For this review, take the finished solid that the model builds, in its own axes (mm). A direction names the side the tool comes from. Give positions to 0.01 mm unless a question says otherwise; leave off trailing zeros. Order: outer loops, then holes, each group sorted by start corner. A loop starts at its lowest first (then second) coordinate and runs counter-clockwise, first axis right, second up. Notation, with made-up numbers: (63, 86.5) -> (70, 86.5) arc R16 ccw to (70, 96.5) -> close; hole circle Ø1 at (51, 11). An arc over 180 degrees is marked (long way). Return JSON: item names as keys, results as strings. Group by question number.
1) For faces 5 (the face through (0, 15, -28)), 6 (the face through (-10.99, 0.99, 8.67)), 7 (the face through (-17, 11, 0)), 8 (the face through (-3, 1, 7)), list the 3-axis set-ups (+Z, -Z, +X, -X, +Y, -Y) from which the entire face can be reached by the end or side of a thin tool; tool diameter is ignored.
2) Add section B-B (z = -35). Give the boundary of the cut face in (x, y), then the cut area to 3 significant figures.
3) To check wall thickness, follow line 1 along Y through (x, z) = (-4, -10); line 2 along Y through (x, z) = (-2.5, -11); line 3 along X through (y, z) = (-3.5, -17). State the ranges of each line that lie inside material, in increasing order.
4) The part is to be moulded in two halves that separate along X. For faces 1 (the face through (0, -25, -12)), 2 (the face through (0, -25, -14)), 3 (the face through (-25, -51, -15)), 4 (the face through (1, 32, 4)), say which applies: released by +X, released by -X, zero draft, split by the parting line, or undercut.
5) Add section A-A (y = -5.5). Give the boundary of the cut face in (x, z).
6) Add section C-C (x = 16). Give the boundary of the cut face in (y, z), then the cut area to 3 significant figures.
7) Insertion check: P1, Ø4, axis at x = 0.5, z = -28, coming from the +Y side; P2, Ø1.6, axis at x = -3.5, y = 37.5, coming from the -Z side; P3, Ø8, axis at y = -10, z = -25.5, coming from the +X side. Each pin has a flat end and moves straight along its axis. Give the tip position at first contact, or say it passes through.
from build123d import *

# Parameters (mm, degrees)
MOTOR_FRONTPLATE_DEPTH           = 2
MOTORKRYBBE_START                = 50
MOTORKRYBBE_DEPTH                = 50
SKYGGE_KAPPE_DEPTH               = 8
SKYGGE_TOPP_DEPTH                = 2
LEDHOLDER_TOPP_DEPTH             = 13
LEDHOLDER_START                  = 13
LEDHOLDER_BUNN_DEPTH             = 13
SKETCH10_R                       = 2.5
LEDHULL_DEPTH                    = 51.950956811
ROTORKAPPE_VEGG_DEPTH            = 20
SKETCH12_R                       = 13
LASERHOLDER_DEPTH                = 4
LASER_HULL_D                     = 6
BUNNPLATE_DEPTH                  = 2
BOSS_EXTRUDE12_DEPTH             = 5
BOSS_EXTRUDE12_DIRECTION_2_REACH = 72.207
LED_START                        = -38
LED_KABELHOLDER_DEPTH            = 38
KABELHOLDER_HULL_REACH           = 73.729
FILLET1_R                        = 5
BOSS_EXTRUDE14_DEPTH             = 5


with BuildPart() as part:
    # Sketch1 → Motor-frontplate (new body)
    with BuildSketch(Plane(origin=(0, 0, 0), x_dir=(1, 0, 0), z_dir=(0, 1, 0))):
        with BuildLine():
            ThreePointArc((-3, 0), (0, 3), (3, 0))
            Line((3, 0), (3, -13.674794331))
            ThreePointArc((3, -13.674794331), (10.908712115, -8.774964387), (14, 0))
            ThreePointArc((14, 0), (0, 14), (-14, 0))
            ThreePointArc((-14, 0), (-10.908712115, -8.774964387), (-3, -13.674794331))
            Line((-3, -13.674794331), (-3, 0))
        make_face()
        with BuildLine():
            Line((14, 0), (24, 0))
            ThreePointArc((24, 0), (0, 24), (-24, 0))
            Line((-24, 0), (-14, 0))
            ThreePointArc((-14, 0), (0, 14), (14, 0))
        make_face()
    extrude(amount=MOTOR_FRONTPLATE_DEPTH)

    # Sketch2 → Motorkrybbe (add)
    with BuildSketch(Plane.XZ.offset(MOTORKRYBBE_START)):
        with BuildLine():
            Line((-12, 0), (-14, 0))
            ThreePointArc((-14, 0), (0, -14), (14, 0))
            Line((14, 0), (12, 0))
            ThreePointArc((12, 0), (0, -12), (-12, 0))
        make_face()
    extrude(amount=-MOTORKRYBBE_DEPTH)

    # Sketch5 → Skygge - Kappe (add)
    with BuildSketch(Plane(origin=(0, 2, 0), x_dir=(1, 0, 0), z_dir=(0, 1, 0))):
        with BuildLine():
            Line((-24, 0), (-22, 0))
            ThreePointArc((-22, 0), (0, 22), (22, 0))
            Line((22, 0), (24, 0))
            ThreePointArc((24, 0), (0, 24), (-24, 0))
        make_face()
    extrude(amount=SKYGGE_KAPPE_DEPTH)

    # Sketch6 → Skygge - Topp (add)
    with BuildSketch(Plane(origin=(0, 10, 0), x_dir=(1, 0, 0), z_dir=(0, 1, 0))):
        with BuildLine():
            Line((-24, 0), (-11, 0))
            ThreePointArc((-11, 0), (0, 11), (11, 0))
            Line((11, 0), (24, 0))
            ThreePointArc((24, 0), (0, 24), (-24, 0))
        make_face()
    extrude(amount=SKYGGE_TOPP_DEPTH)

    # Sketch7 → LEDholder - Topp (add)
    with BuildSketch(Plane(origin=(0, 12, 0), x_dir=(1, 0, 0), z_dir=(0, 1, 0))):
        with BuildLine():
            Line((-4, 12.369316877), (-4, 23.664319132))
            ThreePointArc((-4, 23.664319132), (0, 24), (4, 23.664319132))
            Line((4, 23.664319132), (4, 12.369316877))
            ThreePointArc((4, 12.369316877), (0, 13), (-4, 12.369316877))
        make_face()
    extrude(amount=LEDHOLDER_TOPP_DEPTH)

    # Sketch8 → LEDholder - Bunn (add)
    with BuildSketch(Plane.XZ.offset(LEDHOLDER_START)):
        with BuildLine():
            ThreePointArc((-4, -23.664319132), (0, -24), (4, -23.664319132))
            Line((4, -23.664319132), (4, -13.416407865))
            ThreePointArc((4, -13.416407865), (0, -14), (-4, -13.416407865))
            Line((-4, -13.416407865), (-4, -23.664319132))
        make_face()
    extrude(amount=-LEDHOLDER_BUNN_DEPTH)

    # Sketch10 → LEDhull (cut, through all)
    with BuildSketch(Plane.XZ.offset(13)):
        with Locations(Location((0, -17, 0), (0, 0, 270))):
            Circle(SKETCH10_R)
    extrude(amount=-LEDHULL_DEPTH, mode=Mode.SUBTRACT)

    # Sketch11 → Rotorkappe - Vegg (add)
    with BuildSketch(Plane(origin=(0, 12, 0), x_dir=(1, 0, 0), z_dir=(0, 1, 0))):
        with BuildLine():
            Line((-13, 0), (-11, 0))
            ThreePointArc((-11, 0), (0, 11), (11, 0))
            Line((11, 0), (13, 0))
            ThreePointArc((13, 0), (0, 13), (-13, 0))
        make_face()
    extrude(amount=ROTORKAPPE_VEGG_DEPTH)

    # Sketch12 → Laserholder (add)
    with BuildSketch(Plane(origin=(0, 32, 0), x_dir=(1, 0, 0), z_dir=(0, 1, 0))):
        with Locations(Location((0, 0, 0), (0, 0, 107.920213139))):
            Circle(SKETCH12_R)
    extrude(amount=LASERHOLDER_DEPTH)

    # Laser - hull (through all)
    with Locations(Plane(origin=(0, 36, 0), x_dir=(1, 0, 0), z_dir=(0, 1, 0))):
        with Locations((0, 0)):
            Hole(LASER_HULL_D / 2)

    # Sketch16 → Bunnplate (add)
    with BuildSketch(Plane.XZ.offset(50)):
        with BuildLine():
            Line((-17, -40), (17, -40))
            ThreePointArc((17, -40), (22.656854249, -37.656854249), (25, -32))
            Line((25, -32), (25, 2))
            ThreePointArc((25, 2), (22.656854249, 7.656854249), (17, 10))
            Line((17, 10), (-17, 10))
            ThreePointArc((-17, 10), (-22.656854249, 7.656854249), (-25, 2))
            Line((-25, 2), (-25, -32))
            ThreePointArc((-25, -32), (-22.656854249, -37.656854249), (-17, -40))
        make_face()
    extrude(amount=BUNNPLATE_DEPTH)

    # Sketch19 → Boss-Extrude12 (add)
    with BuildSketch(Plane.XY):
        Polygon((0, -33), (-5, -33), (-5, -30), (-7, -30), (-7, -35), (0, -35), align=None)
    boss_extrude12 = extrude(amount=BOSS_EXTRUDE12_DEPTH)

    # Sketch19 → Boss-Extrude12 direction 2 (add, up to next)
    with BuildSketch(Plane.XY, mode=Mode.PRIVATE) as boss_extrude12_direction_2_sk1:
        Polygon((0, -33), (-5, -33), (-5, -30), (-7, -30), (-7, -35), (0, -35), align=None)
    boss_extrude12_direction_2_tool1 = extrude(boss_extrude12_direction_2_sk1.sketch, amount=-BOSS_EXTRUDE12_DIRECTION_2_REACH, mode=Mode.PRIVATE) - part.part
    boss_extrude12_direction_2 = boss_extrude12_direction_2_tool1.solids().sort_by_distance((-4.25, -33.25, 0))[0]
    add(boss_extrude12_direction_2)

    # Mirror2: Boss-Extrude12, Boss-Extrude12 direction 2 across plane
    add(boss_extrude12.mirror(Plane(origin=(0, -35, -40.002), x_dir=(0, 0, 1), z_dir=(1, 0, 0))))
    add(boss_extrude12_direction_2.mirror(Plane(origin=(0, -35, -40.002), x_dir=(0, 0, 1), z_dir=(1, 0, 0))))

    # Sketch20 → LED - kabelholder (add)
    with BuildSketch(Plane(origin=(0, 25, 0), x_dir=(1, 0, 0), z_dir=(0, 1, 0)).offset(LED_START)):
        with BuildLine():
            Line((4, 23.664319132), (4, 38.664319132))
            Line((4, 38.664319132), (-4, 38.664319132))
            Line((-4, 38.664319132), (-4, 23.664319132))
            ThreePointArc((-4, 23.664319132), (0, 24), (4, 23.664319132))
        make_face()
    extrude(amount=LED_KABELHOLDER_DEPTH)

    # Sketch21 → Kabelholder - hull (cut, up to next)
    with BuildSketch(Plane(origin=(4, 0, 0), x_dir=(0, 0, -1), z_dir=(1, 0, 0)), mode=Mode.PRIVATE) as kabelholder_hull_sk1:
        with BuildLine():
            Line((25.664319132, 15), (30.664319132, 15))
            ThreePointArc((30.664319132, 15), (33.164319132, 17.5), (30.664319132, 20))
            Line((30.664319132, 20), (25.664319132, 20))
            ThreePointArc((25.664319132, 20), (23.164319132, 17.5), (25.664319132, 15))
        make_face()
    kabelholder_hull_tool1 = extrude(kabelholder_hull_sk1.sketch, amount=-KABELHOLDER_HULL_REACH, mode=Mode.PRIVATE) & part.part
    # Sketch21 → Kabelholder - hull (cut, up to next)
    with BuildSketch(Plane(origin=(4, 0, 0), x_dir=(0, 0, -1), z_dir=(1, 0, 0)), mode=Mode.PRIVATE) as kabelholder_hull_sk2:
        with BuildLine():
            ThreePointArc((30.664319132, -3), (33.164319132, -5.5), (30.664319132, -8))
            Line((30.664319132, -8), (25.664319132, -8))
            ThreePointArc((25.664319132, -8), (23.164319132, -5.5), (25.664319132, -3))
            Line((25.664319132, -3), (30.664319132, -3))
        make_face()
    kabelholder_hull_tool2 = extrude(kabelholder_hull_sk2.sketch, amount=-KABELHOLDER_HULL_REACH, mode=Mode.PRIVATE) & part.part
    add(kabelholder_hull_tool1.solids().sort_by_distance((4, 17.5, -28.164319))[0], mode=Mode.SUBTRACT)
    add(kabelholder_hull_tool2.solids().sort_by_distance((4, -5.5, -28.164319))[0], mode=Mode.SUBTRACT)

    # Fillet1
    fillet1_edges = [part.edges().sort_by_distance(p)[0] for p in [
        (0, -13, -38.664319132),
        (0, 25, -38.664319132),
    ]]
    fillet(fillet1_edges, radius=FILLET1_R)

    # Sketch22 → Boss-Extrude14 (add)
    with BuildSketch(Plane(origin=(0, 36, 0), x_dir=(1, 0, 0), z_dir=(0, 1, 0))):
        with BuildLine():
            Line((-3, 0), (-5, 0))
            ThreePointArc((-5, 0), (0, -5), (5, 0))
            Line((5, 0), (3, 0))
            ThreePointArc((3, 0), (0, -3), (-3, 0))
        make_face()
    extrude(amount=BOSS_EXTRUDE14_DEPTH)


solid = part.part
Evaluation:
{
 "1": {"face 5": "+X, -X", "face 6": "+Z, -X, +Y", "face 7": "+Z, -X", "face 8": "+Z"},
 "2": {"outline": "(-24.42, -52) -> (24.42, -52) -> (24.42, -50) -> (-24.42, -50) -> close; (-4, -12.82) -> (4, -12.82) -> (4, 24.82) -> (-4, 24.82) -> close", "area": "399 mm^2"},
 "3": {"line 1": "-52 to -50, -35 to -33, 0 to 2, 32 to 36", "line 2": "-52 to -50, -35 to -33, 0 to 2, 10 to 36", "line 3": "-4 to -2.5, 2.5 to 4"},
 "4": {"face 1": "undercut", "face 2": "split by the parting line", "face 3": "released by -X", "face 4": "undercut"},
 "5": {"outline": "(-14, 0) arc R14 ccw to (-4, -13.42) -> (-4, -23.16) -> (4, -23.16) -> (4, -13.42) arc R14 ccw to (14, 0) -> (12, 0) arc R12 cw to (-12, 0) -> close; (-4, -38.66) -> (4, -38.66) -> (4, -33.16) -> (-4, -33.16) -> close; hole circle Ø5 at (0, -17)"},
 "6": {"outline": "(-52, -40) -> (-50, -40) -> (-50, 10) -> (-52, 10) -> close; (0, -17.89) -> (12, -17.89) -> (12, 0) -> (10, 0) -> (10, -15.1) -> (2, -15.1) -> (2, 0) -> (0, 0) -> close", "area": "194 mm^2"},
 "7": {"P1": "y = 25", "P2": "z = 0", "P3": "x = 4"}
}
